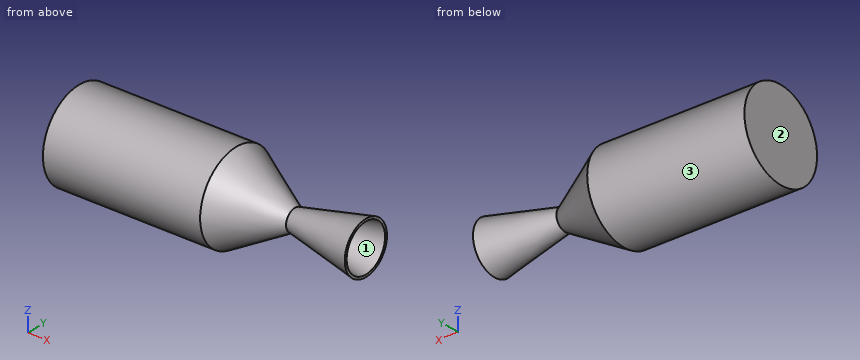
Autodesk Inventor part; units mm, degrees
ref_plane "YZ Plane" through (0, 0, 0) normal (1, 0, 0) x (0, 1, 0)
ref_plane "XZ Plane" through (0, 0, 0) normal (0, 1, 0) x (-1, 0, 0)
ref_plane "XY Plane" through (0, 0, 0) normal (0, 0, 1) x (1, 0, 0)
sketch "Sketch1" plane through (0, 0, 0) normal (0, 0, 1) x (1, 0, 0)
  line L0 (203, 55.5) -> (0, 55.5)
  line L1 (0, 55.5) -> (0, 0)
  line L2 (203, 55.5) -> (280.1, 10.9863)
  line L3 (280.1, 10.9863) -> (374.0063, 30.9467)
  line L4 (-3, 0) -> (-3, 58.5)
  line L5 (-3, 58.5) -> (203.8038, 58.5)
  line L6 (203.8038, 58.5) -> (280.6027, 14.1602)
  line L7 (280.6027, 14.1602) -> (374.0063, 34.0137)
  line L8 (-3, 0) -> (0, 0)
  line L9 (374.0063, 34.0137) -> (374.0063, 30.9467)
  line L10 (-78.4013, 0) -> (449.4075, 0)
  dimension "d11" = 3
revolve "Revolution1" add sketch "Sketch1" angle 360 about axis through (-10, 0, 0) along (1, 0, 0)
properties part number "ESBOÇO 0.1 DO CAD DO MOTOR" material "Steel AISI316"
The model under review builds one solid part; all positions refer to its coordinate system, in mm. Face numbers are marked on the shaded views. Round coordinates to 2 decimals unless told otherwise and drop trailing zeros. Order: outer loops, then holes, each group sorted by start corner. A loop starts at its lowest first (then second) coordinate and runs counter-clockwise, first axis right, second up. Notation, with made-up numbers: (-12, 51) -> (19, 51) arc R6 cw to (19, 62) -> close; hole circle Ø2 at (-39, 0.25). An arc over 180 degrees is marked (long way). Use CSV: the item, a comma, the result in double quotes. Start each with the question number.
(1) Mouldability with a two-part tool opening along Y and no side actions: class the marked faces 1, 2 and 3 as pulls with the +Y half, pulls with the -Y half, needs draft (parallel to the pull), parting line crosses it, or undercut.
(2) Consider section C-C on y = 0. Write out the cut boundary in (x, z).
(3) Consider section B-B on z = -25. State how many separate pieces and enclosed holes the cut face has, and give its area (3 significant figures).
(4) Insertion check: pin 1 (6 mm diameter, centred on x = 48.5, z = -32, fed in from +Y); pin 2 (10 mm diameter, centred on x = 128, y = 8, fed in from -Z); pin 3 (8 mm diameter, centred on x = 336, y = 0, fed in from -Z); pin 4 (8 mm diameter, centred on x = 66.5, z = 2.5, fed in from -Y). Each pin has a flat end and moves straight along its axis. Give the tip position at first contact, or say it passes through.
(5) Consider section A-A on x = 26. Write out the cut boundary in (y, z).
(6) Wall thickness on probe 1 along Z at (x, y) = (154, 0); probe 2 along Z at (x, y) = (109, 6); probe 3 along Y at (x, z) = (13, -42): over which ranges is each line inside the solid? List them lowest first. Write a range as from..to.
Responses:
1,face 1,"undercut"
1,face 2,"needs draft"
1,face 3,"parting line crosses it"
2,outline,"(-3, -58.5) -> (203.8, -58.5) -> (280.6, -14.16) -> (374.01, -34.01) -> (374.01, -30.95) -> (280.1, -10.99) -> (203, -55.5) -> (0, -55.5) -> (0, 55.5) -> (203, 55.5) -> (280.1, 10.99) -> (374.01, 30.95) -> (374.01, 34.01) -> (280.6, 14.16) -> (203.8, 58.5) -> (-3, 58.5) -> close"
3,separate pieces,"2"
3,enclosed holes,"1"
3,area,"2,890 mm²"
4,pin 1,"y = 50.81"
4,pin 2,"z = -58.42"
4,pin 3,"z = -26.79"
4,pin 4,"y = -58.5"
5,outline,"circle Ø117 at (0, 0); hole circle Ø111 at (0, 0)"
6,probe 1,"-58.5..-55.5, 55.5..58.5"
6,probe 2,"-58.19..-55.17, 55.17..58.19"
6,probe 3,"-40.72..-36.28, 36.28..40.72"
